Can you work these out from the model? Positions are in its coordinate system, mm. Face numbers are marked on the shaded views. Round coordinates to 2 decimals unless told otherwise and drop trailing zeros. Write each loop counter-clockwise with the first axis right and the second up, starting at its lowest first coordinate (ties: lowest second). Pieces come first, ordered by that corner, then holes. Notation, with made-up numbers: M 30.5,44 L 78.5,44 A23 ccw 78.5,63 Z; hole C 34,41 d5. An arc over 180 degrees is marked long. Answer in a Markdown table with one row per item. Add a question column.
(1) Suppose I cut it at D-D, the plane y = 0. Write out the boundary of the cut face in (x, z), then the cut area to 3 significant figures.
(2) If we mould it in two halves opening along X, with no side actions, what happens to the marked faces 1, 2 and 3? For each: released by +X, released by -X, zero draft, split by the parting line, or undercut.
(3) Suppose I cut it at C-C, the plane x = 0. Write out the boundary of the cut face in (y, z), then the cut area to 3 significant figures.
(4) If I drill on probe 1 along Y at (x, z) = (57, 23.5); probe 2 along Z at (x, y) = (-21, 35.5); probe 3 along X at (y, z) = (-26, 14), over which ranges is the centre line in solid material (lowest first)?
(5) Suppose I cut it at B-B, the plane z = 33. Count the separate pieces of the cut face and the enclosed holes in it, then the cut area to 3 significant figures.
(6) Suppose I cut it at A-A, the plane y = 57.15. Write out the boundary of the cut face in (x, z), then the cut area to 3 significant figures.
(7) I'm going to push flat-ended pins straight in: pin 1 (3 mm diameter, centred on y = -51.5, z = 7, fed in from -X); pin 2 (10 mm diameter, centred on x = 11.5, y = -29.5, fed in from +Z); pin 3 (1 mm diameter, centred on y = 46, z = 14, fed in from -X); pin 4 (6 mm diameter, centred on x = -30, y = 47.5, fed in from -Z). Where does each tip first touch, or does it pass through?
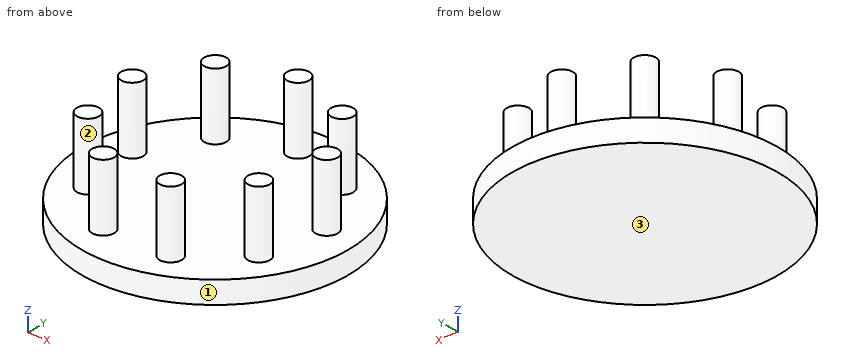
Autodesk Inventor part; units mm, degrees
ref_plane "YZ Plane" through (0, 0, 0) normal (1, 0, 0) x (0, 1, 0)
ref_plane "XZ Plane" through (0, 0, 0) normal (0, 1, 0) x (-1, 0, 0)
ref_plane "XY Plane" through (0, 0, 0) normal (0, 0, 1) x (1, 0, 0)
sketch "Sketch1" plane through (0, 0, 0) normal (0, 0, 1) x (1, 0, 0)
  circle A0 centre (0, 0) radius 76.2
  dimension "d0" = 152.4
extrude "Extrusion1" add sketch "Sketch1" along normal blind 12.7
sketch "Sketch2" plane through (0, 0, 12.7) normal (0, 0, 1) x (1, 0, 0)
  circle A0 centre (0, 0) radius 76.2
  circle A1 centre (0, 57.15) radius 6.35
  dimension "d3" = 12.7
  dimension "d4" = 57.15
extrude "Extrusion2" add sketch "Sketch2" along normal blind 38.1 contours A1
pattern_circular "Circular Pattern1" count 9 over 360 about axis through (0, 0, 0) along (0, 0, 1) of "Extrusion2"
properties part number "holder"
Calculated:
| question | item | result |
|---|---|---|
| 1 | outline | M -76.2,0 L 76.2,0 L 76.2,12.7 L -76.2,12.7 Z |
| 1 | area | 1,940 mm² |
| 2 | face 1 | split by the parting line |
| 2 | face 2 | undercut |
| 2 | face 3 | zero draft |
| 3 | outline | M -76.2,0 L 76.2,0 L 76.2,12.7 L 63.5,12.7 L 63.5,50.8 L 50.8,50.8 L 50.8,12.7 L -76.2,12.7 Z |
| 3 | area | 2,420 mm² |
| 4 | probe 1 | 3.61 to 16.23 |
| 4 | probe 2 | 0 to 12.7 |
| 4 | probe 3 | -55.3 to -43.69, 43.69 to 55.3 |
| 5 | separate pieces | 9 |
| 5 | enclosed holes | 0 |
| 5 | area | 1,140 mm² |
| 6 | outline | M -50.4,0 L 50.4,0 L 50.4,12.7 L 6.35,12.7 L 6.35,50.8 L -6.35,50.8 L -6.35,12.7 L -50.4,12.7 Z |
| 6 | area | 1,760 mm² |
| 7 | pin 1 | x = -57.5 |
| 7 | pin 2 | z = 12.7 |
| 7 | pin 3 | x = -42.85 |
| 7 | pin 4 | z = 0 |
